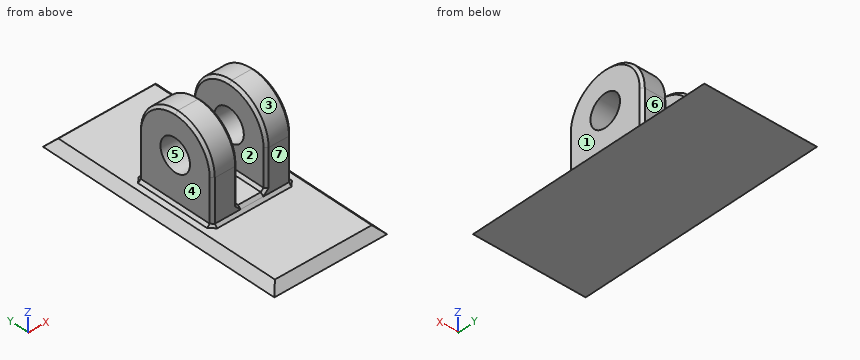
from build123d import *

# Parameters (mm, degrees)
SKETCH1_W               = 21.25
SKETCH1_H               = 47
BOSS_EXTRUDE1_DEPTH     = 1.5
CHAMFER1_SIZE           = 1.5
SKETCH2_W               = 15
SKETCH2_H               = 15
BOSS_EXTRUDE2_DEPTH     = 16
SKETCH3_W               = 5.3
SKETCH3_H               = 15
CUT_EXTRUDE1_DEPTH      = 15
CUT_EXTRUDE2_DEPTH      = 35.453093112
CUT_EXTRUDE2_DEPTH_BACK = 35.453093112
SKETCH4_R               = 3
FILLET1_R               = 7.5
CHAMFER2_SIZE           = 0.5


with BuildPart() as part:
    # Sketch1 → Boss-Extrude1 (new body)
    with BuildSketch(Plane.XY):
        Rectangle(SKETCH1_W, SKETCH1_H)
    extrude(amount=BOSS_EXTRUDE1_DEPTH)

    # Chamfer1
    chamfer1_edges = [part.edges().sort_by_distance(p)[0] for p in [
        (0, -23.5, 1.5),
        (-10.625, 0, 1.5),
        (0, 23.5, 1.5),
        (10.625, 0, 1.5),
    ]]
    chamfer(chamfer1_edges, length=CHAMFER1_SIZE - 0.0001)  # a hair under: the kernel refuses the full size

    # Sketch2 → Boss-Extrude2 (add)
    with BuildSketch(Plane.XY.offset(1.5)):
        Rectangle(SKETCH2_W, SKETCH2_H)
    extrude(amount=BOSS_EXTRUDE2_DEPTH)

    # Sketch3 → Cut-Extrude1 (cut)
    with BuildSketch(Plane.XY.offset(17.5)):
        Rectangle(SKETCH3_W, SKETCH3_H)
    extrude(amount=-CUT_EXTRUDE1_DEPTH, mode=Mode.SUBTRACT)

    # Sketch4 → Cut-Extrude2 (cut, two sides: drawn at the far end of the back side and taken through both)
    with BuildSketch(Plane.ZY.offset(7.5).offset(-CUT_EXTRUDE2_DEPTH_BACK)):
        with Locations((10, 0)):
            Circle(SKETCH4_R)
    extrude(amount=CUT_EXTRUDE2_DEPTH + CUT_EXTRUDE2_DEPTH_BACK, mode=Mode.SUBTRACT)

    # Fillet1
    fillet1_edges = [part.edges().sort_by_distance(p)[0] for p in [
        (5.075, -7.5, 17.5),
        (5.075, 7.5, 17.5),
        (-5.075, 7.5, 17.5),
        (-5.075, -7.5, 17.5),
    ]]
    fillet(fillet1_edges, radius=FILLET1_R - 0.0001)  # a hair under: the kernel refuses the full size

    # Chamfer2
    chamfer2_edges = [part.edges().sort_by_distance(p)[0] for p in [
        (7.5, 0, 1.5),
        (0, 7.5, 1.5),
        (-7.5, 0, 1.5),
        (0, -7.5, 1.5),
        (2.65, 0, 2.5),
        (2.65, 7.5, 6.25005),
        (0, -7.5, 2.5),
        (2.65, -7.5, 6.25005),
        (-2.65, 0, 2.5),
        (-2.65, -7.5, 6.25005),
        (0, 7.5, 2.5),
        (-2.65, 7.5, 6.25005),
        (7.5, 7.5, 5.75005),
        (7.5, -7.5, 5.75005),
        (7.5, 5.303330148, 15.303330148),
        (7.5, -5.303330148, 15.303330148),
        (-7.5, -7.5, 5.75005),
        (2.65, 5.303330148, 15.303330148),
        (2.65, -5.303330148, 15.303330148),
        (-7.5, 7.5, 5.75005),
        (-7.5, -5.303330148, 15.303330148),
        (-7.5, 5.303330148, 15.303330148),
        (-2.65, -5.303330148, 15.303330148),
        (-2.65, 5.303330148, 15.303330148),
    ]]
    chamfer(chamfer2_edges, length=CHAMFER2_SIZE - 0.0001)  # a hair under: the kernel refuses the full size


solid = part.part
Check sheet for the modelled part. Datum: model origin and axes. Units: mm. Face numbers are marked on the shaded views. A direction names the side the tool comes from. Round coordinates to 2 decimals unless told otherwise and drop trailing zeros. Loops run counter-clockwise (first coordinate to the right, second up) from the corner with the lowest first, then second, coordinate; pieces in that order, holes last. Notation, with made-up numbers: M -5.5,-13.5 L 51.5,-13.5 A18 cw 51.5,6.5 Z; hole C 26.5,62 d1. An arc over 180 degrees is marked long. One line per question, with ' | ' between items. Start each with the question number.
Item 1: Set-up check for the marked faces 1, 2 and 3: record each of +Z, -Z, +X, -X, +Y, -Y from which the full face is reachable in a straight line by a thin tool's end or side.
Item 2: Gauge pin test, flat ends, axial feed: pin 1 Ø4 at (y, z) = (-2.5, 7) entering from +X; pin 2 Ø7 at (y, z) = (2.5, 12) entering from -X; pin 3 Ø8 at (x, y) = (2, -7) entering from +Z; pin 4 Ø2.5 at (x, z) = (-1, 6) entering from +Y. Record the tip position at first contact, or that the pin passes through.
Item 3: Section check D-D (y = 0.5). State how many separate pieces and enclosed holes the cut face has, and give its area (3 significant figures).
Item 4: Section check A-A (z = 6.25). Record the boundary of the cut face in (x, y), and give its area (4 significant figures).
Item 5: Scan lines: probe 1 along X at (y, z) = (0, 15.5); probe 2 along Y at (x, z) = (-4.05, 10); probe 3 along Z at (x, y) = (-4.25, 0). Record each from-to range of solid material in increasing order.
Item 6: Release check for a two-part mould opening along Y. For the marked faces 4, 5, 6 and 7 record: released by +Y, released by -Y, zero draft, split by the parting line, or undercut.
Worked out:
1) face 1: +Z, +X, +Y, -Y | face 2: +Z, +Y, -Y | face 3: +Z, +X, -X, -Y
2) pin 1: x = 7.5 | pin 2: x = -7.5 | pin 3: z = 16.8 | pin 4: through
3) separate pieces: 3 | enclosed holes: 0 | area: 133 mm^2
4) outline: M -7.5,-7 L -7,-7.5 L -3.15,-7.5 L -2.65,-7 L -2.65,7 L -3.15,7.5 L -7,7.5 L -7.5,7 Z; M 2.65,-7 L 3.15,-7.5 L 7,-7.5 L 7.5,-7 L 7.5,7 L 7,7.5 L 3.15,7.5 L 2.65,7 Z | area: 144.5 mm^2
5) probe 1: -7.5 to -2.65, 2.65 to 7.5 | probe 2: -7.5 to -3, 3 to 7.5 | probe 3: 0 to 7, 13 to 17.5
6) face 4: zero draft | face 5: undercut | face 6: released by +Y | face 7: released by -Y
